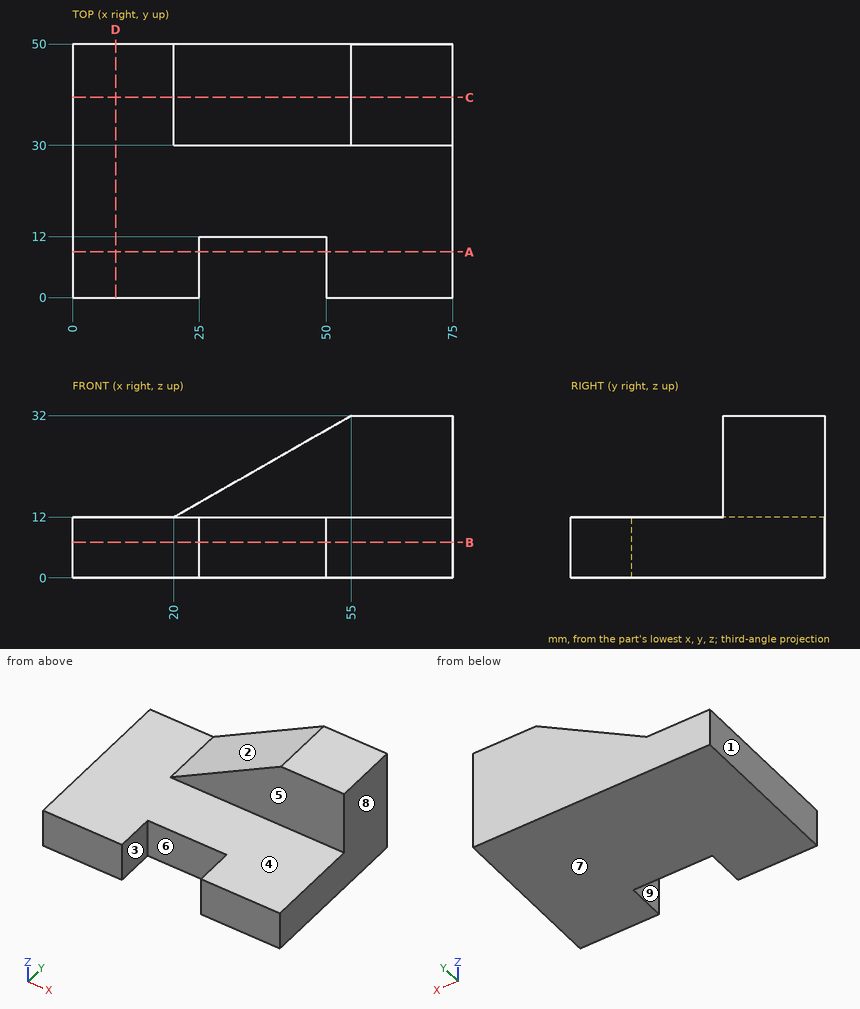
Can you work these out from the drawing? Everything is in mm from the part's minimum corner. A direction names the side the tool comes from. Give positions to 0.01 mm unless a question says otherwise; leave off trailing zeros. Order: outer loops, then holes, each group sorted by start corner. A loop starts at its lowest first (then second) coordinate and runs counter-clockwise, first axis right, second up. Notation, with made-up numbers: M -28,69.25 L 4,69.25 A22 cw 4,96.25 Z; hole C 67.5,2.5 d2. An arc over 180 degrees is marked long. One line per item, written item: value.
Item 1: If we section it at B-B on z = 7: Write out the boundary of the cut face in (x, y).
Verdict:
outline: M 0,0 L 25,0 L 25,12 L 50,12 L 50,0 L 75,0 L 75,50 L 0,50 Z
Item 2: For the marked faces 1, 2, 3, 4 and 5, which set-ups out of +Z, -Z, +X, -X, +Y, -Y let a thin tool reach every point of the face, with its end or its side?
Verdict:
face 1: +Z, -Z, -X, +Y, -Y
face 2: +Z, -X, +Y, -Y
face 3: +Z, -Z, -Y
face 4: +Z, -X, -Y
face 5: +Z, +X, -X, -Y
Item 3: For pin 1 (10 mm diameter, centred on x = 52, z = 19, fed in from -Y); pin 2 (8 mm diameter, centred on x = 41, y = 17, fed in from +Z); pin 3 (6 mm diameter, centred on x = 33, z = 6, fed in from -Y), each with a flat end and sliding along its axis, tell me the tip position at first contact or that it passes through.
Verdict:
pin 1: y = 30
pin 2: z = 12
pin 3: y = 12
Item 4: If we section it at C-C on y = 39.5: Write out the boundary of the cut face in (x, z).
Verdict:
outline: M 0,0 L 75,0 L 75,32 L 55,32 L 20,12 L 0,12 Z
Item 5: If we section it at D-D on x = 8.5: Write out the boundary of the cut face in (y, z), and give its area (3 significant figures).
Verdict:
outline: M 0,0 L 50,0 L 50,12 L 0,12 Z
area: 600 mm2
Item 6: If we section it at A-A on y = 9: Write out the boundary of the cut face in (x, z).
Verdict:
outline: M 0,0 L 25,0 L 25,12 L 0,12 Z; M 50,0 L 75,0 L 75,12 L 50,12 Z
Item 7: If we mould it in two halves opening along X, with no side actions, what happens to the marked faces 6, 7, 8 and 9? For each: pulls with the +X half, pulls with the -X half, needs draft (parallel to the pull), parting line crosses it, or undercut.
Verdict:
face 6: undercut
face 7: needs draft
face 8: pulls with the +X half
face 9: undercut
Item 8: Please list where these lines run through material, in increasing order: line 1 (Z direction, x = 11.5, y = 35.5); line 2 (Y direction, x = 32.5, z = 18.5); line 3 (X direction, y = 42.5, z = 17.5) (3 decimals).
Verdict:
line 1: 0 to 12
line 2: 30 to 50
line 3: 29.625 to 75
